Check sheet for the modelled part. Datum: model origin and axes. Units: mm. A direction names the side the tool comes from. Give positions to 0.01 mm unless a question says otherwise; leave off trailing zeros. Write each loop counter-clockwise with the first axis right and the second up, starting at its lowest first coordinate (ties: lowest second). Pieces come first, ordered by that corner, then holes. Notation, with made-up numbers: M -19,69 L -13,69 A12 ccw -13,79 Z; hole C 49.5,-13 d1. An arc over 180 degrees is marked long. Use CSV: the item, a comma, the result in double quotes. Start each with the question number.
1. Cross-section at A-A, the plane y = -7.75. Enter the section's corners in (x, z), and give its area (3 significant figures).
2. Scan line: line 1 (Y direction, x = -11, z = 15) (3 decimals). Record every from-to range of solid material in increasing order.
3. Cross-section at C-C, the plane x = 11. Enter the section's corners in (y, z) (3 decimals).
4. Depth check by flat-ended pin: P1, Ø2.5, axis at x = -19, z = 12.5, coming from the -Y side (3 decimals); P2, Ø10, axis at x = 20, y = -13, coming from the -Z side; P3, Ø10, axis at y = -13.5, z = 18, coming from the +X side; P4, Ø10, axis at y = -14.5, z = -15.5, coming from the -X side. Enter the tip coordinate at first touch or a pass-through.
5. Mould release check, pull along X, two halves, no side actions. Record for faces 1 (the face through (24.696, -11.224, 0.356)), 2 (the face through (-25.4, -2, 0)), 3 (the face through (0, -5, 25.4)), 4 (the face through (-12, -3.175, 0)): +X half, -X half, draft (parallel to the pull), parting line (faces both ways), or undercut.
6. Access from +Z, -Z, +X, -X, +Y, -Y to the whole of each face (thin tool, end or side, straight path). Record for faces 5 (the face through (-24.715, -11.001, 0.356)), 6 (the face through (-7.054, -11.224, 0.356)).
7. Cross-section at D-D, the plane y = -17.25. Enter the section's corners in (x, z), and give its area (3 significant figures).
from build123d import *

# Parameters (mm, degrees)
SKETCH1_W           = 50.8
SKETCH1_H           = 50.8
BOSS_EXTRUDE1_DEPTH = 3.175
BOSS_EXTRUDE2_DEPTH = 50.8
LPATTERN1_COUNT     = 7
LPATTERN1_PITCH     = 7.9375


with BuildPart() as part:
    # Sketch1 → Boss-Extrude1 (new body)
    with BuildSketch(Plane(origin=(0, 0, 0), x_dir=(1, 0, 0), z_dir=(0, 1, 0))):
        Rectangle(SKETCH1_W, SKETCH1_H)
    extrude(amount=-BOSS_EXTRUDE1_DEPTH)

    # Sketch2 → Boss-Extrude2 (add, through all)
    with BuildSketch(Plane.XY.offset(25.4)):
        Polygon((-25.4, -3.175), (-24.01062, -19.05), (-23.61438, -19.05), (-22.225, -3.175), align=None)
    boss_extrude2 = extrude(amount=-BOSS_EXTRUDE2_DEPTH)

    # LPattern1: Boss-Extrude2 ×7
    with Locations(*[(i * LPATTERN1_PITCH, 0, 0) for i in range(1, LPATTERN1_COUNT)]):
        add(boss_extrude2)


solid = part.part
Worked answers:
1,outline,"M -25,-25.4 L -22.63,-25.4 L -22.63,25.4 L -25,25.4 Z; M -17.06,-25.4 L -14.69,-25.4 L -14.69,25.4 L -17.06,25.4 Z; M -9.12,-25.4 L -6.75,-25.4 L -6.75,25.4 L -9.12,25.4 Z; M -1.19,-25.4 L 1.19,-25.4 L 1.19,25.4 L -1.19,25.4 Z; M 6.75,-25.4 L 9.12,-25.4 L 9.12,25.4 L 6.75,25.4 Z; M 14.69,-25.4 L 17.06,-25.4 L 17.06,25.4 L 14.69,25.4 Z; M 22.63,-25.4 L 25,-25.4 L 25,25.4 L 22.63,25.4 Z"
1,area,"844 mm^2"
2,line 1,"y = -3.175 to 0"
3,outline,"M -3.175,-25.4 L 0,-25.4 L 0,25.4 L -3.175,25.4 Z"
4,P1,"stops at y = -3.175"
4,P2,"stops at z = -25.4"
4,P3,"stops at x = 24.93"
4,P4,"stops at x = -24.85"
5,face 1,"+X half"
5,face 2,"-X half"
5,face 3,"draft"
5,face 4,"undercut"
6,face 5,"+Z, -Z, -X, -Y"
6,face 6,"+Z, -Z, -Y"
7,outline,"M -24.17,-25.4 L -23.46,-25.4 L -23.46,25.4 L -24.17,25.4 Z; M -16.23,-25.4 L -15.52,-25.4 L -15.52,25.4 L -16.23,25.4 Z; M -8.29,-25.4 L -7.58,-25.4 L -7.58,25.4 L -8.29,25.4 Z; M -0.36,-25.4 L 0.36,-25.4 L 0.36,25.4 L -0.36,25.4 Z; M 7.58,-25.4 L 8.29,-25.4 L 8.29,25.4 L 7.58,25.4 Z; M 15.52,-25.4 L 16.23,-25.4 L 16.23,25.4 L 15.52,25.4 Z; M 23.46,-25.4 L 24.17,-25.4 L 24.17,25.4 L 23.46,25.4 Z"
7,area,"253 mm^2"
